Read the model definition and answer for the solid it produces. Units are mm, in the model's axes. A direction names the side the tool comes from. Give positions to 0.01 mm unless a question says otherwise; leave off trailing zeros. Order: outer loops, then holes, each group sorted by start corner. A loop starts at its lowest first (then second) coordinate and runs counter-clockwise, first axis right, second up. Notation, with made-up numbers: M -26.75,-3 L 11.25,-3 A19 cw 11.25,18 Z; hole C -3,-11 d5. An arc over 180 degrees is marked long. Write item = value, one per line. Start each with the question number.
from build123d import *

# Parameters (mm, degrees)
SKETCH1_W           = 30
SKETCH1_H           = 30.88
BOSS_EXTRUDE1_DEPTH = 5.44
SKETCH2_W           = 19
SKETCH2_H           = 12
CUT_EXTRUDE1_DEPTH  = 44.395483636
CAVITY1_OUTLINE_W   = 10
CAVITY1_OUTLINE_H   = 5.44
CAVITY1_DEPTH       = 5.44
CAVITY1_START       = 25.44
CAVITY1_2_OUTLINE_W = 10
CAVITY1_2_OUTLINE_H = 5.44
CAVITY1_2_DEPTH     = 5.44


# Read off the part's stored shape, not the designer's step: Cavity1
with BuildPart() as part:
    # Sketch1 → Boss-Extrude1 (new body)
    with BuildSketch(Plane.XY):
        with Locations((15, 15.44)):
            Rectangle(SKETCH1_W, SKETCH1_H)
    extrude(amount=BOSS_EXTRUDE1_DEPTH)

    # Sketch2 → Cut-Extrude1 (cut, through all)
    with BuildSketch(Plane(origin=(0, 0, 0), x_dir=(-1, 0, 0), z_dir=(0, 0, -1))):
        with Locations((-15, 15.44)):
            Rectangle(SKETCH2_W, SKETCH2_H)
    extrude(amount=-CUT_EXTRUDE1_DEPTH, mode=Mode.SUBTRACT)

    # Cavity1 outline → Cavity1 (cut)
    with BuildSketch(Plane(origin=(0, 0, 0), x_dir=(1, 0, 0), z_dir=(0, 1, 0))):
        with Locations((15, -2.72)):
            Rectangle(CAVITY1_OUTLINE_W, CAVITY1_OUTLINE_H)
    extrude(amount=CAVITY1_DEPTH, mode=Mode.SUBTRACT)

    # Cavity1 2 outline → Cavity1 2 (cut)
    with BuildSketch(Plane(origin=(0, 0, 0), x_dir=(1, 0, 0), z_dir=(0, 1, 0)).offset(CAVITY1_START)):
        with Locations((15, -2.72)):
            Rectangle(CAVITY1_2_OUTLINE_W, CAVITY1_2_OUTLINE_H)
    extrude(amount=CAVITY1_2_DEPTH, mode=Mode.SUBTRACT)


solid = part.part
1) Find section C-C on z = 2.1. Determine the outline of the cut face in (x, y).
2) Find the intervals of material crossed by probe 1 along Y at (x, z) = (8.75, 2.8); probe 2 along Y at (x, z) = (15, 4.8); probe 3 along X at (y, z) = (14.5, 1.4), in increasing order. Write a range as [from, to].
3) Find section B-B on x = 14.75. Determine the outline of the cut face in (y, z), plus the area to 3 significant figures.
4) Each of these flat-tipped pins is pushed along its axis until it touches: P1, Ø4, axis at x = 9, y = 17.5, coming from the -Z side; P2, Ø1.6, axis at x = 17.5, z = 3, coming from the +Y side. Where does it stop, or does it pass through?
5) For faces 5 (the face through (20, 3, 3)), 6 (the face through (15, 25.44, 3)), 7 (the face through (5.5, 15, 3)), 8 (the face through (25, 0, 3)), determine the directions among +Z, -Z, +X, -X, +Y, -Y from which every point of the face is accessible in a straight line to the end or side of a thin tool.
6) Find section A-A on y = 20. Determine the outline of the cut face in (x, z), plus the area to 3 significant figures.
7) For a pull along X with two mould halves and no side action, classify faces 1 (the face through (25, 30.88, 3)), 2 (the face through (0, 15, 3)), 3 (the face through (30, 15, 3)), 4 (the face through (10, 28, 3)) as pulls with the +X half, pulls with the -X half, needs draft (parallel to the pull), parting line crosses it, or undercut.
Numbers:
q1.outline = M 0,0 L 10,0 L 10,5.44 L 20,5.44 L 20,0 L 30,0 L 30,30.88 L 20,30.88 L 20,25.44 L 10,25.44 L 10,30.88 L 0,30.88 Z; hole M 5.5,9.44 L 24.5,9.44 L 24.5,21.44 L 5.5,21.44 Z
q2.probe_1 = [0, 9.44], [21.44, 30.88]
q2.probe_2 = [5.44, 9.44], [21.44, 25.44]
q2.probe_3 = [0, 5.5], [24.5, 30]
q3.outline = M 5.44,0 L 9.44,0 L 9.44,5.44 L 5.44,5.44 Z; M 21.44,0 L 25.44,0 L 25.44,5.44 L 21.44,5.44 Z
q3.area = 43.5 mm2
q4.P1 = through
q4.P2 = 25.44
q5.face_5 = +Z, -Z, -Y
q5.face_6 = +Z, -Z, +Y
q5.face_7 = +Z, -Z
q5.face_8 = +Z, -Z, +X, -X, -Y
q6.outline = M 0,0 L 5.5,0 L 5.5,5.44 L 0,5.44 Z; M 24.5,0 L 30,0 L 30,5.44 L 24.5,5.44 Z
q6.area = 59.8 mm2
q7.face_1 = needs draft
q7.face_2 = pulls with the -X half
q7.face_3 = pulls with the +X half
q7.face_4 = undercut
